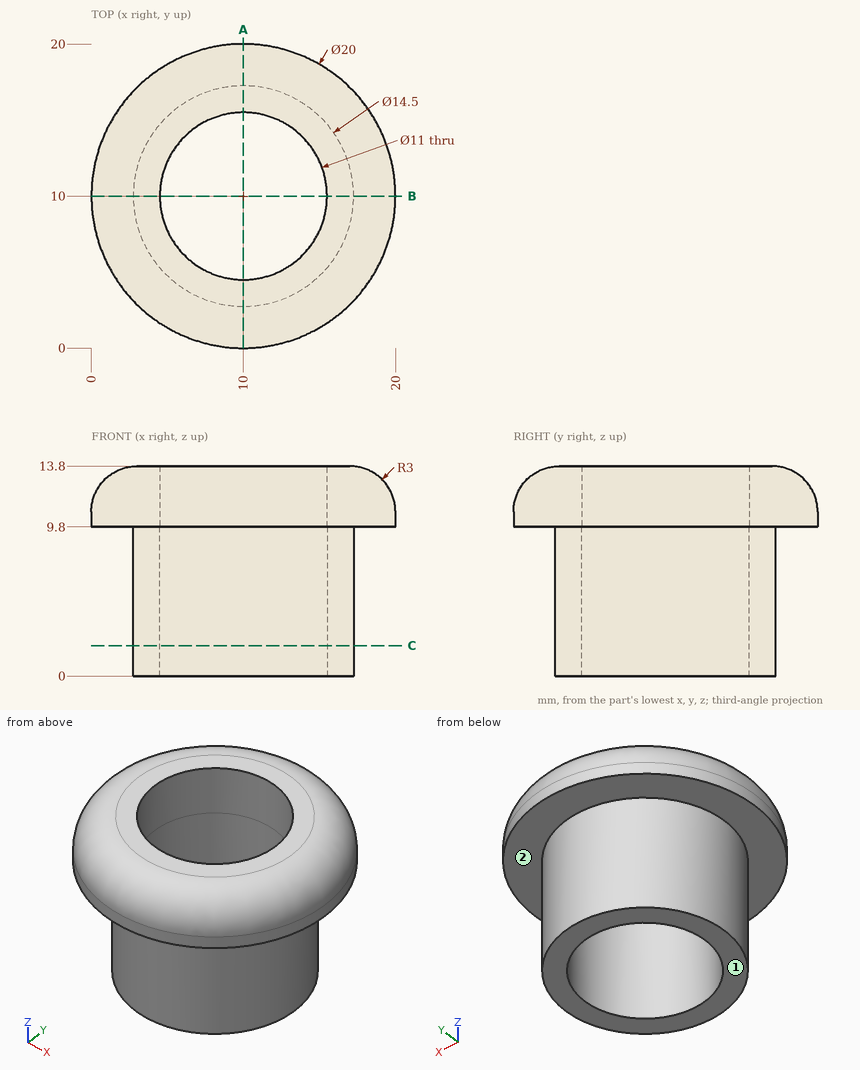
Study the drawing (mm; zero at the part's minimum x, y, z) and answer. A direction names the side the tool comes from. Give positions to 0.01 mm unless a question says otherwise; leave off trailing zeros. Write each loop counter-clockwise with the first axis right and the second up, starting at its lowest first coordinate (ties: lowest second). Pieces come first, ordered by that corner, then holes.
Item 1: Flat-ended cylindrical pins translate along their axes: P1, Ø6, axis at x = 13.5, z = 5, coming from the -Y side; P2, Ø6, axis at y = 10, z = 5, coming from the -X side; P3, Ø6, axis at y = 2.5, z = 6.5, coming from the +X side; P4, Ø1.5, axis at x = 7.5, y = 14.5, coming from the +Z side. Find the tip coordinate at first contact, or state that the pin passes through.
Item 2: Section A-A, the plane x = 10 is taken. Write down the section's boundary in (y, z).
Item 3: Find the intervals of material crossed by line 1 along Y through (x, z) = (10, 10.9); line 2 along X through (y, z) = (10.25, 2); line 3 along Y through (x, z) = (10, 3.5), in increasing order.
Item 4: Section C-C, the plane z = 2 is taken. Write down the section's boundary in (x, y), plus the area to 3 significant figures.
Item 5: Which of the six approach directions +Z, -Z, +X, -X, +Y, -Y give full straight-line access (tool end or side, diameter ignored) to the marked faces 1 and 2?
Completed:
1. P1: stops at y = 2.77
1. P2: stops at x = 2.75
1. P3: stops at x = 15.68
1. P4: stops at z = 13.8
2. outline: (0, 9.8) - (2.75, 9.8) - (2.75, 0) - (4.5, 0) - (4.5, 13.8) - (3, 13.8) arc R3 ccw to (0, 10.8) - close; (15.5, 0) - (17.25, 0) - (17.25, 9.8) - (20, 9.8) - (20, 10.8) arc R3 ccw to (17, 13.8) - (15.5, 13.8) - close
3. line 1: y = 0 to 4.5, 15.5 to 20
3. line 2: x = 2.75 to 4.51, 15.49 to 17.25
3. line 3: y = 2.75 to 4.5, 15.5 to 17.25
4. outline: circle Ø14.5 at (10, 10); hole circle Ø11 at (10, 10)
4. area: 70.1 mm2
5. face 1: -Z, +X, -X, +Y, -Y
5. face 2: -Z
